from build123d import *

# Parameters (mm, degrees)
SKETCH1_W               = 203.2
SKETCH1_H               = 279.4
BOSS_EXTRUDE1_DEPTH     = 6.35
CUT_EXTRUDE1_START      = -7.35
SKETCH2_R               = 2.54
SKETCH2_W               = 25.4
SKETCH2_H               = 25.4
CUT_EXTRUDE1_DEPTH      = 8.35
LPATTERN1_COUNT         = 2
LPATTERN1_PITCH         = 152.4
LPATTERN1_COUNT_DIR2    = 2
LPATTERN1_PITCH_DIR2    = 152.4
SKETCH3_W               = 44.45
SKETCH3_H               = 88.9
SKETCH3_R               = 10.16
CUT_EXTRUDE2_DEPTH      = 1
CUT_EXTRUDE2_DEPTH_BACK = 7.35


with BuildPart() as part:
    # Sketch1 → Boss-Extrude1 (new body)
    with BuildSketch(Plane(origin=(0, 0, 0), x_dir=(1, 0, 0), z_dir=(0, 1, 0))):
        Rectangle(SKETCH1_W, SKETCH1_H)
    extrude(amount=BOSS_EXTRUDE1_DEPTH)

    # Sketch2 → Cut-Extrude1 (cut)
    with BuildSketch(Plane(origin=(0, 6.35, 0), x_dir=(1, 0, 0), z_dir=(0, 1, 0)).offset(CUT_EXTRUDE1_START)):
        with Locations((-55.8038, 76.2)):
            Circle(SKETCH2_R)
        with Locations((-76.2, 55.8038)):
            Circle(SKETCH2_R)
        with Locations((-96.5962, 76.2)):
            Circle(SKETCH2_R)
        with Locations((-76.2, 96.5962)):
            Circle(SKETCH2_R)
        with Locations((-76.2, 76.2)):
            Rectangle(SKETCH2_W, SKETCH2_H)
    cut_extrude1 = extrude(amount=CUT_EXTRUDE1_DEPTH, mode=Mode.SUBTRACT)

    # LPattern1: Cut-Extrude1 2 × 2
    with Locations(*[(i * LPATTERN1_PITCH, 0, j * LPATTERN1_PITCH_DIR2) for i in range(LPATTERN1_COUNT) for j in range(LPATTERN1_COUNT_DIR2) if (i, j) != (0, 0)]):
        add(cut_extrude1, mode=Mode.SUBTRACT)

    # Sketch3 → Cut-Extrude2 (cut, two sides)
    with BuildSketch(Plane(origin=(0, 6.35, 0), x_dir=(1, 0, 0), z_dir=(0, 1, 0))) as cut_extrude2_sk:
        with Locations((0, 92.71)):
            Rectangle(SKETCH3_W, SKETCH3_H)
        with Locations((0, 76.2)):
            Circle(SKETCH3_R, mode=Mode.SUBTRACT)
        with Locations((0, -53.086)):
            Rectangle(SKETCH3_W, SKETCH3_H)
        with Locations((0, -76.2)):
            Circle(SKETCH3_R, mode=Mode.SUBTRACT)
        with Locations((0, 76.2)):
            Circle(SKETCH3_R)
        with Locations((0, -76.2)):
            Circle(SKETCH3_R)
    extrude(amount=CUT_EXTRUDE2_DEPTH, mode=Mode.SUBTRACT)
    extrude(cut_extrude2_sk.sketch, amount=-CUT_EXTRUDE2_DEPTH_BACK, mode=Mode.SUBTRACT)


solid = part.part
Source: CAD feature listing. Evaluate the final solid. Frame: model axes, mm. A direction names the side the tool comes from. Round coordinates to 2 decimals unless told otherwise and drop trailing zeros. Loops run counter-clockwise (first coordinate to the right, second up) from the corner with the lowest first, then second, coordinate; pieces in that order, holes last. Notation, with made-up numbers: M 63,23 L 98,23 A16 cw 98,30 Z; hole C 18,52.25 d4. An arc over 180 degrees is marked long. Return JSON: item names as keys, results as strings. Group by question number.
1. Mould query, pull axis X, two halves, no side actions, for faces 3 (the face through (101.6, 3, 2)), 4 (the face through (63.5, 3, 76)), 5 (the face through (-1, 6.35, -2)), 6 (the face through (-88.9, 3, 76)). Classes: released by +X, released by -X, zero draft, split by the parting line, or undercut.
2. Section query C-C on x = 67.5. Output: boundary loops of the cut face in (y, z).
3. Pin query (flat end, axial travel): pin 1 (4.5 mm diameter, centred on x = 76.2, z = 55.8, fed in from -Y); pin 2 (8 mm diameter, centred on x = 55.8, z = 76.2, fed in from +Y). Return the tip coordinate at first contact, or that it passes through.
4. Reachability of faces 1 (the face through (-1, 0, -2)), 2 (the face through (-63.5, 3, -76)) from +Z, -Z, +X, -X, +Y, -Y: full face, straight path, thin tool, end or side. Return the list, or none.
5. Section query B-B on x = -18.5. Output: boundary loops of the cut face in (y, z).
6. Section query D-D on y = 2.25. State how many separate pieces and enclosed holes the cut face has, and give its area (3 significant figures).
7. Section query A-A on z = 18. Output: boundary loops of the cut face in (x, y) (3 decimals), and give its area (3 significant figures).
8. Material intervals for line 1 along Z through (x, y) = (2, 1.75); line 2 along X through (y, z) = (6, -82.5) (3 decimals); line 3 along X through (y, z) = (6, 95) (3 decimals), sorted ascending. Write a range as from..to.
Checks:
{
 "1": {"face 3": "released by +X", "face 4": "undercut", "face 5": "zero draft", "face 6": "undercut"},
 "2": {"outline": "M 0,-139.7 L 6.35,-139.7 L 6.35,-88.9 L 0,-88.9 Z; M 0,-63.5 L 6.35,-63.5 L 6.35,63.5 L 0,63.5 Z; M 0,88.9 L 6.35,88.9 L 6.35,139.7 L 0,139.7 Z"},
 "3": {"pin 1": "passes through", "pin 2": "stops at y = 6.35"},
 "4": {"face 1": "+Z, -Z, +X, -X, -Y", "face 2": "+Y, -Y"},
 "5": {"outline": "M 0,-139.7 L 6.35,-139.7 L 6.35,-137.16 L 0,-137.16 Z; M 0,-48.26 L 6.35,-48.26 L 6.35,8.64 L 0,8.64 Z; M 0,97.54 L 6.35,97.54 L 6.35,139.7 L 0,139.7 Z"},
 "6": {"separate pieces": "1", "enclosed holes": "22", "area": "46,000 mm²"},
 "7": {"outline": "M -101.6,0 L -22.225,0 L -22.225,6.35 L -101.6,6.35 Z; M 22.225,0 L 101.6,0 L 101.6,6.35 L 22.225,6.35 Z", "area": "1,010 mm²"},
 "8": {"line 1": "z = -139.7..-137.16, -48.26..8.64, 97.54..139.7", "line 2": "x = -101.6..-88.9, -63.5..-22.225, 22.225..63.5, 88.9..101.6", "line 3": "x = -101.6..-78.176, -74.224..-22.225, 22.225..74.224, 78.176..101.6"}
}
